from build123d import *

# Parameters (mm, degrees)
SKETCH1_W           = 3.17
SKETCH1_H           = 3.17
BOSS_EXTRUDE1_DEPTH = 3.17


with BuildPart() as part:
    # Sketch1 → Boss-Extrude1 (new body)
    with BuildSketch(Plane(origin=(0, 0, 0), x_dir=(0, 0, -1), z_dir=(1, 0, 0))):
        with Locations((13.415, 31.355)):
            Rectangle(SKETCH1_W, SKETCH1_H)
        with Locations((1.585, 31.355)):
            Rectangle(SKETCH1_W, SKETCH1_H)
        with Locations((1.585, 1.585)):
            Rectangle(SKETCH1_W, SKETCH1_H)
        with Locations((13.415, 1.585)):
            Rectangle(SKETCH1_W, SKETCH1_H)
        Polygon((11.83, 3.17), (11.83, 29.77), (11.83, 32.94), (3.17, 32.94), (3.17, 29.77), (3.17, 3.17), (3.17, 0), (11.83, 0), align=None)
    extrude(amount=BOSS_EXTRUDE1_DEPTH)


solid = part.part
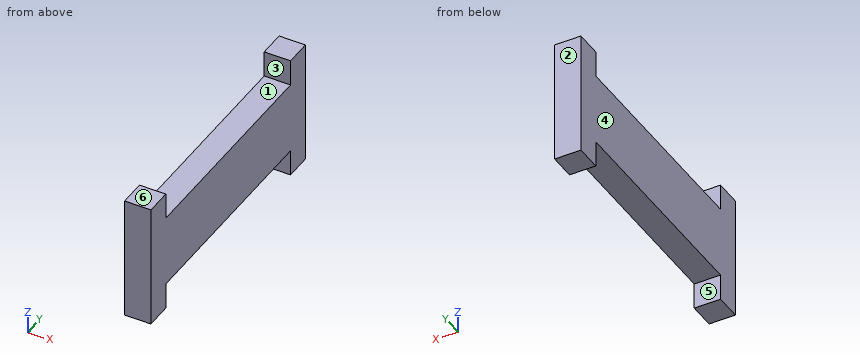
The model under review builds one solid part; all positions refer to its coordinate system, in mm. Face numbers are marked on the shaded views. A direction names the side the tool comes from. Coordinates: 2 decimals unless noted, no trailing zeros. Write each loop counter-clockwise with the first axis right and the second up, starting at its lowest first coordinate (ties: lowest second). Pieces come first, ordered by that corner, then holes. Notation, with made-up numbers: M 37,50.5 L 85,50.5 A36 cw 85,86.5 Z; hole C 7,5 d10. An arc over 180 degrees is marked long. Put each result on its own line as item: value.
1) Add section A-A on z = -14. Give the boundary of the cut face in (x, y), then the cut area to 3 significant figures.
Computed:
outline: M 0,0 L 3.17,0 L 3.17,3.17 L 0,3.17 Z; M 0,29.77 L 3.17,29.77 L 3.17,32.94 L 0,32.94 Z
area: 20.1 mm2
2) Add section C-C on y = 8.5. Give the boundary of the cut face in (x, z), then the cut area to 3 significant figures.
Computed:
outline: M 0,-11.83 L 3.17,-11.83 L 3.17,-3.17 L 0,-3.17 Z
area: 27.5 mm2
3) Wall thickness on probe 1 along Y at (x, z) = (1.45, -1); probe 2 along Z at (x, y) = (1.7, 13): over which ranges is each line inside the solid? List them lowest first. Write a range as [from, to].
Computed:
probe 1: y = [0, 3.17], [29.77, 32.94]
probe 2: z = [-11.83, -3.17]
4) Clearance check with flat-ended pins moving along their axes: pin 1 Ø1.6 at (x, y) = (1.5, 23) entering from +Z; pin 2 Ø1.5 at (x, y) = (2, 4.5) entering from -Z. State where each tip first meets the part, or that it passes through.
Computed:
pin 1: stops at z = -3.17
pin 2: stops at z = -11.83
5) Add section B-B on x = 1.55. Give the boundary of the cut face in (y, z), then the cut area to 3 significant figures.
Computed:
outline: M 0,-15 L 3.17,-15 L 3.17,-11.83 L 29.77,-11.83 L 29.77,-15 L 32.94,-15 L 32.94,0 L 29.77,0 L 29.77,-3.17 L 3.17,-3.17 L 3.17,0 L 0,0 Z
area: 325 mm2
6) Draft analysis for pull direction Y (two halves, no side actions). For the marked faces 1, 2, 3 and 4, state which applies: released by +Y, released by -Y, zero draft, split by the parting line, or undercut.
Computed:
face 1: undercut
face 2: released by +Y
face 3: undercut
face 4: zero draft
7) For the marked faces 5 and 6, list the 3-axis set-ups (+Z, -Z, +X, -X, +Y, -Y) from which the entire face can be reached by the end or side of a thin tool; tool diameter is ignored.
Computed:
face 5: -Z, +X, -X
face 6: +Z, +X, -X, +Y, -Y
